from build123d import *
from build123d.topology import SkipClean

# Parameters (mm, degrees)
SKETCH_1_R                      = 5
SKETCH_1_R_2                    = 2.5
EXTRUDE_1_DEPTH                 = 10
EXTRUDE_1_2_DEPTH               = 10
EXTRUDE_1_3_DEPTH               = 10
EXTRUDE_1_4_DEPTH               = 10
EXTRUDE_1_5_DEPTH               = 10
EXTRUDE_1_6_DEPTH               = 10
EXTRUDE_2_DEPTH                 = 6
EXTRUDE_4_DEPTH                 = 6
CUT_EXTRUDE_1_DEPTH             = 4
SKETCH_5_R                      = 3.75
SKETCH_5_R_2                    = 2.5
EXTRUDE_3_DEPTH                 = 2
CUT_EXTRUDE_2_DEPTH             = 4
CUT_EXTRUDE_3_DEPTH             = 8
SKETCH_11_R                     = 2.5
EXTRUDE_9_DEPTH                 = 2
AUFSATZ_LINEAR_AUSTRAGEN1_DEPTH = 6
SKIZZE4_W                       = 5
SKIZZE4_H                       = 59.806963929
SCHNITT_LINEAR_AUSTRAGEN1_DEPTH = 8
SCHNITT_LINEAR_AUSTRAGEN2_DEPTH = 8
SCHNITT_LINEAR_AUSTRAGEN3_DEPTH = 8
SCHNITT_LINEAR_AUSTRAGEN6_DEPTH = 8
SCHNITT_LINEAR_START            = -4
SCHNITT_LINEAR_AUSTRAGEN7_DEPTH = 4


with BuildPart() as part:
    # Sketch 1 → Extrude 1 (new body)
    with BuildSketch(Plane.XY):
        with Locations((-12.085916667, 4.294857344)):
            Circle(SKETCH_1_R)
        with Locations((-12.085916667, 4.294857344)):
            Circle(SKETCH_1_R_2, mode=Mode.SUBTRACT)
    extrude(amount=EXTRUDE_1_DEPTH)



with BuildPart() as body_2:
    # Sketch 1 → Extrude 1 2 (new body)
    with BuildSketch(Plane.XY):
        with Locations((-38.24886757, -21.86809356)):
            Circle(SKETCH_1_R)
        with Locations((-38.24886757, -21.86809356)):
            Circle(SKETCH_1_R_2, mode=Mode.SUBTRACT)
    extrude(amount=EXTRUDE_1_2_DEPTH)


with BuildPart() as body_3:
    # Sketch 1 → Extrude 1 3 (new body)
    with BuildSketch(Plane.XY):
        with Locations((14.077034237, -21.86809356)):
            Circle(SKETCH_1_R)
        with Locations((14.077034237, -21.86809356)):
            Circle(SKETCH_1_R_2, mode=Mode.SUBTRACT)
    extrude(amount=EXTRUDE_1_3_DEPTH)


with BuildPart() as body_4:
    # Sketch 1 → Extrude 1 4 (new body)
    with BuildSketch(Plane.XY):
        with Locations((-38.24886757, -81.86809356)):
            Circle(SKETCH_1_R)
        with Locations((-38.24886757, -81.86809356)):
            Circle(SKETCH_1_R_2, mode=Mode.SUBTRACT)
    extrude(amount=EXTRUDE_1_4_DEPTH)


with BuildPart() as body_5:
    # Sketch 1 → Extrude 1 5 (new body)
    with BuildSketch(Plane.XY):
        with Locations((14.077034237, -81.86809356)):
            Circle(SKETCH_1_R)
        with Locations((14.077034237, -81.86809356)):
            Circle(SKETCH_1_R_2, mode=Mode.SUBTRACT)
    extrude(amount=EXTRUDE_1_5_DEPTH)


with BuildPart() as body_6:
    # Sketch 1 → Extrude 1 6 (new body)
    with BuildSketch(Plane.XY):
        with Locations((-12.085916667, -108.031044464)):
            Circle(SKETCH_1_R)
        with Locations((-12.085916667, -108.031044464)):
            Circle(SKETCH_1_R_2, mode=Mode.SUBTRACT)
    extrude(amount=EXTRUDE_1_6_DEPTH)


with BuildPart() as part_1:
    add(part.part)

    add(body_2.part)  # Extrude 2 merges body 2
    # Sketch 3 → Extrude 2 (add)
    with BuildSketch(Plane(origin=(0, 0, 0), x_dir=(-1, 0, 0), z_dir=(0, 0, -1))):
        Polygon((12.085916667, 4.294857344), (15.621450572, 7.83039125), (41.784401476, -18.332559654), (34.713333665, -25.403627466), (8.550382761, 0.759323438), align=None)
    extrude(amount=-EXTRUDE_2_DEPTH)


    add(body_3.part)  # Extrude 4 merges body 3
    # Sketch 9 → Extrude 4 (add)
    with BuildSketch(Plane(origin=(0, 0, 0), x_dir=(-1, 0, 0), z_dir=(0, 0, -1))):
        Polygon((-14.077034237, -21.86809356), (-17.612568143, -18.332559654), (8.550382761, 7.83039125), (15.621450572, 0.759323438), (-10.541500331, -25.403627466), align=None)
    extrude(amount=-EXTRUDE_4_DEPTH)

    # Sketch 4 → Cut-Extrude 1 (cut)
    with BuildSketch(Plane.XY.offset(6)):
        Polygon((-13.85368362, 6.062624297), (-10.318149714, 2.527090391), (-36.481100617, -23.635860513), (-40.016634523, -20.100326607), align=None)
    extrude(amount=-CUT_EXTRUDE_1_DEPTH, mode=Mode.SUBTRACT)

    # Sketch 5 → Extrude 3 (add)
    with BuildSketch(Plane(origin=(0, 0, 0), x_dir=(-1, 0, 0), z_dir=(0, 0, -1))):
        with Locations((12.969800143, 5.178740821)):
            Circle(SKETCH_5_R)
        with Locations(Location((38.24886757, -21.86809356, 0), (0, 0, 45))):
            Circle(SKETCH_5_R_2)
    extrude(amount=-EXTRUDE_3_DEPTH)

    # Sketch 4_2 → Cut-Extrude 2 (cut)
    with BuildSketch(Plane.XY.offset(6)):
        Polygon((-13.85368362, 6.062624297), (-10.318149714, 2.527090391), (-36.481100617, -23.635860513), (-40.016634523, -20.100326607), align=None)
    extrude(amount=CUT_EXTRUDE_2_DEPTH, mode=Mode.SUBTRACT)

    # Sketch 10 → Cut-Extrude 3 (cut)
    with BuildSketch(Plane.XY.offset(10)):
        Polygon((14.077034237, -21.86809356), (12.309267284, -23.635860513), (-13.85368362, 2.527090391), (-12.085916667, 4.294857344), (-10.318149714, 6.062624297), (15.84480119, -20.100326607), align=None)
    extrude(amount=-CUT_EXTRUDE_3_DEPTH, mode=Mode.SUBTRACT)

    # Sketch 11 → Extrude 9 (add)
    with BuildSketch(Plane(origin=(0, 0, 0), x_dir=(-1, 0, 0), z_dir=(0, 0, -1))):
        with Locations((-14.077034237, -21.86809356)):
            Circle(SKETCH_11_R)
    extrude(amount=-EXTRUDE_9_DEPTH)


    add(body_4.part)  # Aufsatz-Linear austragen1 merges body 4

    add(body_5.part)  # Aufsatz-Linear austragen1 merges body 5

    add(body_6.part)  # Aufsatz-Linear austragen1 merges body 6
    # Skizze2 → Aufsatz-Linear austragen1 (add)
    with BuildSketch(Plane(origin=(0, 0, 0), x_dir=(-1, 0, 0), z_dir=(0, 0, -1))):
        with BuildLine():
            Line((-19.077034237, -21.86809356), (-19.077034237, -82.509912102))
            ThreePointArc((-19.077034237, -82.509912102), (-18.955201687, -83.290446679), (-18.601294786, -83.996723751))
            Line((-18.601294786, -83.996723751), (-17.963462032, -85.013833377))
            Line((-17.963462032, -85.013833377), (8.547769183, -111.563962859))
            Line((8.547769183, -111.563962859), (15.62406415, -111.563962859))
            Line((15.62406415, -111.563962859), (41.784377989, -85.403650953))
            Line((41.784377989, -85.403650953), (43.24886757, -81.86809356))
            Line((43.24886757, -81.86809356), (43.24886757, -21.86809356))
            Line((43.24886757, -21.86809356), (33.24886757, -23.939161372))
            Line((33.24886757, -23.939161372), (33.24886757, -81.86809356))
            Line((33.24886757, -81.86809356), (12.085916667, -103.031044464))
            Line((12.085916667, -103.031044464), (-9.077034237, -81.86809356))
            Line((-9.077034237, -81.86809356), (-9.077034237, -23.939161372))
            Line((-9.077034237, -23.939161372), (-19.077034237, -21.86809356))
        make_face()
    extrude(amount=-AUFSATZ_LINEAR_AUSTRAGEN1_DEPTH)

    # Skizze4 → Schnitt-Linear austragen1 (cut)
    with SkipClean():  # the faces are left unmerged after this step: merging them gives an invalid solid
        with BuildSketch(Plane.XY.offset(10)):
            with Locations((14.077034237, -51.964611596)):
                Rectangle(SKIZZE4_W, SKIZZE4_H)
        extrude(amount=-SCHNITT_LINEAR_AUSTRAGEN1_DEPTH, mode=Mode.SUBTRACT)

    # Skizze5 → Schnitt-Linear austragen2 (cut)
    with SkipClean():  # the faces are left unmerged after this step: merging them gives an invalid solid
        with BuildSketch(Plane.XY.offset(10)):
            Polygon((-38.24886757, -81.86809356), (-35.74886757, -81.86809356), (-35.74886757, -21.86809356), (-40.74886757, -21.86809356), (-40.74886757, -81.86809356), align=None)
        extrude(amount=-SCHNITT_LINEAR_AUSTRAGEN2_DEPTH, mode=Mode.SUBTRACT)

    # Skizze6 → Schnitt-Linear austragen3 (cut)
    with SkipClean():  # the faces are left unmerged after this step: merging them gives an invalid solid
        with BuildSketch(Plane.XY.offset(10)):
            Polygon((-12.815807368, -107.346754652), (13.705977842, -80.78605569), (16.182665193, -83.259114477), (-10.339120017, -109.819813439), align=None)
        extrude(amount=-SCHNITT_LINEAR_AUSTRAGEN3_DEPTH, mode=Mode.SUBTRACT)

    # Skizze8 → Schnitt-Linear austragen6 (cut)
    with SkipClean():  # the faces are left unmerged after this step: merging them gives an invalid solid
        with BuildSketch(Plane.XY.offset(10)):
            Polygon((-37.36882645, -81.283668587), (-11.186213036, -107.466282), (-13.66108677, -109.941155734), (-39.843700184, -83.758542321), align=None)
        extrude(amount=-SCHNITT_LINEAR_AUSTRAGEN6_DEPTH, mode=Mode.SUBTRACT)

    # Skizze10 → Schnitt-Linear austragen7 (cut)
    with SkipClean():  # the faces are left unmerged after this step: merging them gives an invalid solid
        with BuildSketch(Plane.XY.offset(6).offset(SCHNITT_LINEAR_START)):
            with BuildLine():
                Line((-11.940605405, -108.220674369), (-13.66108677, -109.941155734))
                Line((-13.66108677, -109.941155734), (-14.125547986, -109.476694519))
                ThreePointArc((-14.125547986, -109.476694519), (-12.311454238, -110.52085024), (-10.339260555, -109.819673108))
                Line((-10.339260555, -109.819673108), (-11.940605405, -108.220674369))
            make_face()
            with BuildLine():
                Line((-12.962669252, -105.689825784), (-12.061327377, -106.591167659))
                Line((-12.061327377, -106.591167659), (-11.174544611, -105.703083773))
                ThreePointArc((-11.174544611, -105.703083773), (-12.067381012, -105.531113179), (-12.962669252, -105.689825784))
            make_face()
            with BuildLine():
                Line((-39.843700184, -83.758542321), (-37.953251423, -81.86809356))
                Line((-37.953251423, -81.86809356), (-40.74886757, -81.86809356))
                ThreePointArc((-40.74886757, -81.86809356), (-40.46969232, -83.01610812), (-39.694517625, -83.907724879))
                Line((-39.694517625, -83.907724879), (-39.843700184, -83.758542321))
            make_face()
            with BuildLine():
                Line((-36.784401476, -81.86809356), (-35.907648891, -82.744846145))
                ThreePointArc((-35.907648891, -82.744846145), (-35.78888315, -82.313600744), (-35.74886757, -81.86809356))
                Line((-35.74886757, -81.86809356), (-36.784401476, -81.86809356))
            make_face()
            with BuildLine():
                Line((14.789603319, -81.86809356), (16.165610117, -83.242084387))
                ThreePointArc((16.165610117, -83.242084387), (16.471970531, -82.585226846), (16.577034237, -81.86809356))
                Line((16.577034237, -81.86809356), (14.789603319, -81.86809356))
            make_face()
            with BuildLine():
                Line((11.739718918, -82.755199583), (12.625525252, -81.86809356))
                Line((12.625525252, -81.86809356), (11.577034237, -81.86809356))
                ThreePointArc((11.577034237, -81.86809356), (11.61804173, -82.319043502), (11.739718918, -82.755199583))
            make_face()
            with BuildLine():
                Line((19.077034237, -82.509912102), (19.077034237, -81.86809356))
                ThreePointArc((19.077034237, -81.86809356), (18.956650141, -82.958666175), (18.601294786, -83.996723751))
                ThreePointArc((18.601294786, -83.996723751), (18.955201687, -83.290446679), (19.077034237, -82.509912102))
            make_face()
        extrude(amount=SCHNITT_LINEAR_AUSTRAGEN7_DEPTH, mode=Mode.SUBTRACT)


solid = part_1.part
Part model, mm, in its own coordinate system. A direction names the side the tool comes from. Coordinates: 2 decimals unless noted, no trailing zeros. Loops run counter-clockwise (first coordinate to the right, second up) from the corner with the lowest first, then second, coordinate; pieces in that order, holes last. Notation, with made-up numbers: M 69.5,43.25 L 77.5,43.25 A29 cw 77.5,74.25 Z; hole C -16.5,12.25 d1. An arc over 180 degrees is marked long. Use a Markdown table: item, result. Add a question column.
Q1. Cut at C-C (z = 4.5). Give the number of separate pieces and of enclosed holes in the cut face, and give its area (3 significant figures).
Q2. Which spindle directions (+Z, -Z, +X, -X, +Y, -Y) get a long thin tool onto all of the face, cutting with end or side? Do faces 4 (the flat face through (3, -98, 6)), 5 (the flat face through (4, -6, 6)), 6 (the flat face through (-1.65, -13.21, 2.96)), 7 (the flat face through (3.11, -96.35, 4.28)). Say none if no direction does.
Q3. Mould opens along Y. For faces 1 (the flat face through (-12, -111, 10)), 2 (the cylindrical face through (9.227, -80.654, 7.972)), 3 (the flat face through (0.12, -94.39, 4.28)) say: +Y half, -Y half, draft (parallel to the pull), parting line (faces both ways), or undercut.
Q4. Probe L1, parallel to X at y = -62, z = 3.25; L2, parallel to Y at x = -8, z = 4.75; L3, parallel to Y at x = -29, z = 3.5. List the from-to ranges inside material, lowest first.
Q5. Cut at B-B (x = -5.5). Write the cut outline in (y, z), and give its area (3 significant figures).
Q6. Pin check, flat tips, straight feed: P1, Ø8, axis at x = 4.5, y = 0, coming from the +Z side; P2, Ø3, axis at x = -23.5, z = 4.5, coming from the -Y side; P3, Ø4, axis at x = -10, z = 3.5, coming from the +Y side; P4, Ø5, axis at x = -1.5, z = 2, coming from the -Y side. Stop position of each tip, or through.
Q7. Cut at A-A (y = -73). Write the cut outline in (x, z).
Worked out:
| question | item | result |
|---|---|---|
| 1 | separate pieces | 2 |
| 1 | enclosed holes | 2 |
| 1 | area | 1,340 mm2 |
| 2 | face 4 | +Z, +X, -Y |
| 2 | face 5 | +Z, +X, +Y |
| 2 | face 6 | +Z, -Z |
| 2 | face 7 | +Z |
| 3 | face 1 | draft |
| 3 | face 2 | undercut |
| 3 | face 3 | undercut |
| 4 | L1 | x = -43.25 to -40.75, -35.75 to -33.25, 9.08 to 11.58, 16.58 to 19.08 |
| 4 | L2 | y = -111.02 to -107.48, -102.52 to -98.95, -6.86 to -3.33, 3.74 to 7.28 |
| 4 | L3 | y = -98.19 to -94.6, -89.65 to -86.12, -19.69 to -16.15, -9.08 to -5.55 |
| 5 | outline | M -108.51,0 L -96.45,0 L -96.45,6 L -100.02,6 L -100.02,2 L -104.97,2 L -104.97,6 L -108.51,6 Z; M -9.36,0 L 4.78,0 L 4.78,6 L 1.24,6 L 1.24,2 L -5.83,2 L -5.83,6 L -9.36,6 Z |
| 5 | area | 109 mm2 |
| 6 | P1 | stops at z = 6 |
| 6 | P2 | stops at y = -105.19 |
| 6 | P3 | stops at y = 9.29 |
| 6 | P4 | stops at y = -107.01 |
| 7 | outline | M -43.25,0 L -33.25,0 L -33.25,6 L -35.75,6 L -35.75,2 L -40.75,2 L -40.75,6 L -43.25,6 Z; M 9.08,0 L 19.08,0 L 19.08,6 L 16.58,6 L 16.58,2 L 11.58,2 L 11.58,6 L 9.08,6 Z |
